Geometry: see drawing. Coordinates: mm, zero at the bounding-box minimum. Give positions to 0.01 mm unless a question says otherwise; leave off trailing zeros. Loops run counter-clockwise (first coordinate to the right, second up) from the corner with the lowest first, then second, coordinate; pieces in that order, holes last. Notation, with made-up numbers: (66, 55.5) - (83, 55.5) arc R15 ccw to (83, 75.5) - close; hole circle Ø4 at (-29, 8). An arc over 180 degrees is marked (long way). Use one line per item in the form item = value.
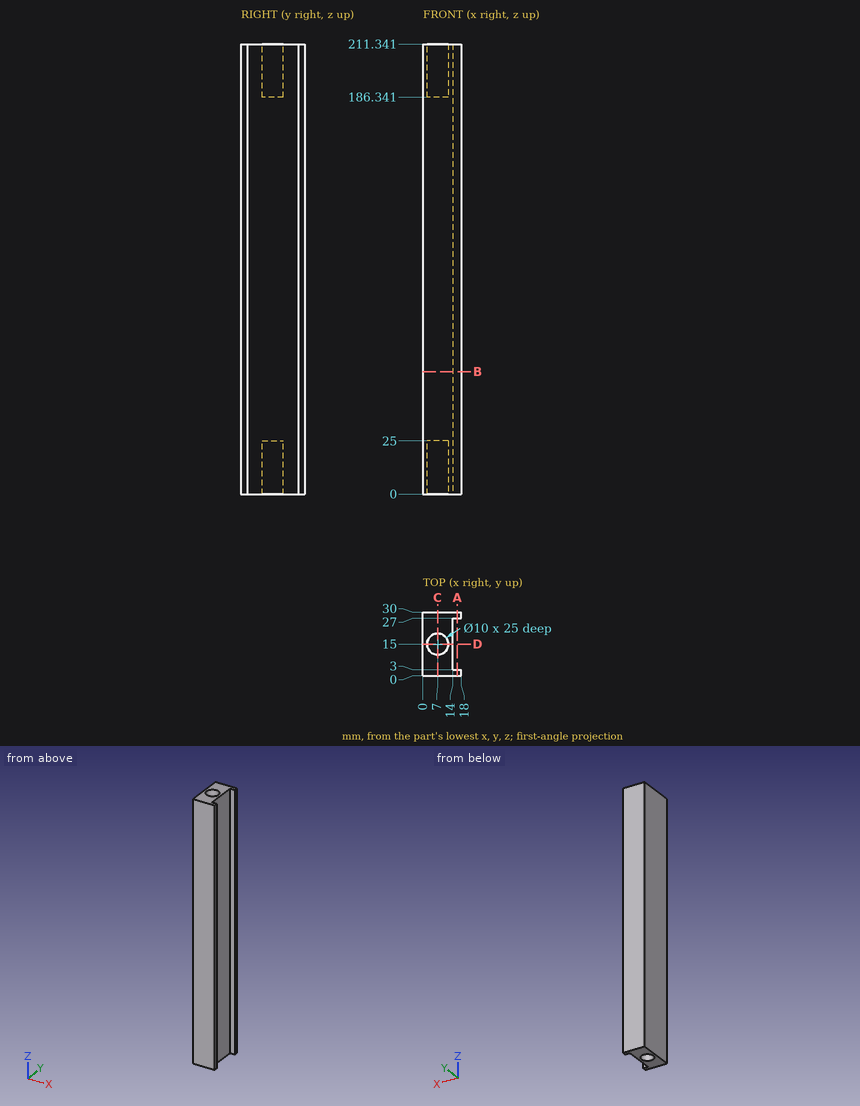
(1) Cut plane A-A (x = 16.25). Return the cut outline in (y, z).
Solution:
outline = (0, 0) - (3, 0) - (3, 211.34) - (0, 211.34) - close; (27, 0) - (30, 0) - (30, 211.34) - (27, 211.34) - close
(2) Cut plane D-D (y = 15). Return the cut outline in (x, z), plus the area to 3 significant figures.
Solution:
outline = (0, 0) - (2, 0) - (2, 25) - (12, 25) - (12, 0) - (14, 0) - (14, 211.34) - (12, 211.34) - (12, 186.34) - (2, 186.34) - (2, 211.34) - (0, 211.34) - close
area = 2,460 mm2
(3) Pin query (flat end, axial travel): P1, Ø7, axis at y = 13.5, z = 70.5, coming from the +X side; P2, Ø5, axis at x = 7, y = 16, coming from the +Z side. Return the tip coordinate at first contact, or that it passes through.
Solution:
P1 = 14
P2 = 186.34
(4) Cut plane B-B (z = 57.5). Return the cut outline in (x, y), plus the area to 3 significant figures.
Solution:
outline = (0, 0) - (18, 0) - (18, 3) - (14, 3) - (14, 27) - (18, 27) - (18, 30) - (0, 30) - close
area = 444 mm2
(5) Cut plane C-C (x = 7). Return the cut outline in (y, z).
Solution:
outline = (0, 0) - (10, 0) - (10, 25) - (20, 25) - (20, 0) - (30, 0) - (30, 211.34) - (20, 211.34) - (20, 186.34) - (10, 186.34) - (10, 211.34) - (0, 211.34) - close
(6) Material intervals for L1, parallel to X at y = 15, z = 7.25; L2, parallel to Y at x = 7, z = 20.25; L3, parallel to Y at x = 16, z = 200, sorted ascending. Write a range as from..to.
Solution:
L1 = 0..2, 12..14
L2 = 0..10, 20..30
L3 = 0..3, 27..30
